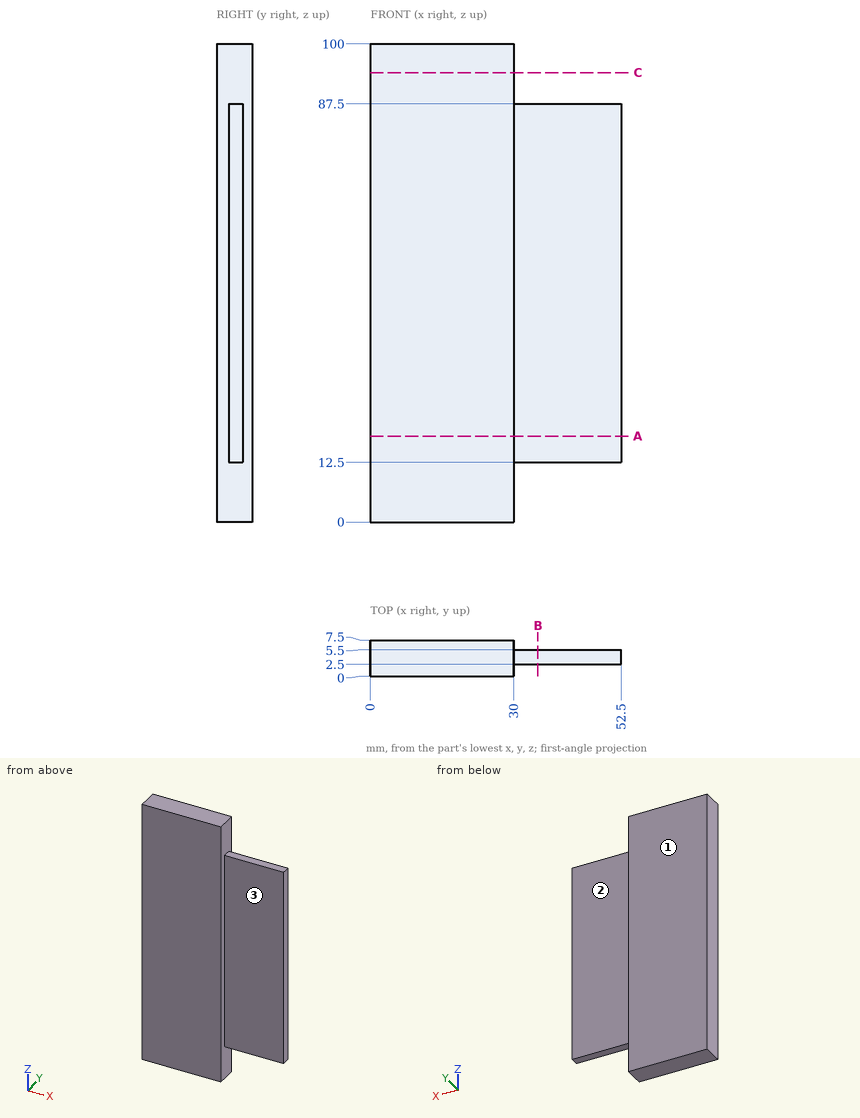
Geometry check sheet. Reference: drawing and pictorial views, mm from the part's lowest x, y, z. A direction names the side the tool comes from. Coordinates: 2 decimals unless noted, no trailing zeros. Write each loop counter-clockwise with the first axis right and the second up, starting at its lowest first coordinate (ties: lowest second). Pieces come first, ordered by that corner, then holes. Notation, with made-up numbers: M 11,-11.75 L 34,-11.75 A8 ccw 34,0.25 Z; hole C -12.75,68.25 d11. An arc over 180 degrees is marked long. Use one line per item in the form item = value.
Item 1: Sectioned sample at A-A, the plane z = 18. Record the cut outline in (x, y).
Answer below:
outline = M 0,0 L 30,0 L 30,2.5 L 52.5,2.5 L 52.5,5.5 L 30,5.5 L 30,7.5 L 0,7.5 Z
Item 2: Sectioned sample at C-C, the plane z = 94. Record the cut outline in (x, y), and give its area (3 significant figures).
Answer below:
outline = M 0,0 L 30,0 L 30,7.5 L 0,7.5 Z
area = 225 mm^2
Item 3: Gauge pin test, flat ends, axial feed: pin 1 Ø4 at (x, z) = (35.5, 14) entering from -Y; pin 2 Ø2 at (x, y) = (44, 1) entering from -Z; pin 3 Ø2.5 at (x, y) = (46, 4) entering from +Z; pin 4 Ø3.5 at (x, y) = (39.5, 3.5) entering from -Z. Record the tip position at first contact, or that the pin passes through.
Answer below:
pin_1 = 2.5
pin_2 = through
pin_3 = 87.5
pin_4 = 12.5
Item 4: Material ranges on L1, parallel to Y at x = 42, z = 21.5; L2, parallel to X at y = 1.25, z = 46; L3, parallel to Z at x = 49, y = 4, recorded low to high. Write a range as from..to.
Answer below:
L1 = 2.5..5.5
L2 = 0..30
L3 = 12.5..87.5
Item 5: Set-up check for the marked faces 1, 2 and 3: record each of +Z, -Z, +X, -X, +Y, -Y from which the full face is reachable in a straight line by a thin tool's end or side.
Answer below:
face_1 = +Z, -Z, +X, -X, +Y
face_2 = +Z, -Z, +X, +Y
face_3 = +Z, -Z, +X, -Y
Item 6: Sectioned sample at B-B, the plane x = 35. Record the cut outline in (y, z).
Answer below:
outline = M 2.5,12.5 L 5.5,12.5 L 5.5,87.5 L 2.5,87.5 Z
